from build123d import *

# Parameters (mm, degrees)
SKETCH1_W           = 100
SKETCH1_H           = 30
SKETCH1_R           = 1.5
BOSS_EXTRUDE1_DEPTH = 2
SKETCH2_W           = 1
SKETCH2_H           = 30
BOSS_EXTRUDE3_DEPTH = 50
FILLET2_R           = 1
SKETCH3_R           = 1.5
CUT_EXTRUDE1_DEPTH  = 10
FILLET3_R           = 10
BOSS_EXTRUDE4_DEPTH = 2


with BuildPart() as part:
    # Sketch1 → Boss-Extrude1 (new body)
    with BuildSketch(Plane.XY):
        with Locations((50, 15)):
            Rectangle(SKETCH1_W, SKETCH1_H)
        with Locations((10, 15)):
            Circle(SKETCH1_R, mode=Mode.SUBTRACT)
    extrude(amount=BOSS_EXTRUDE1_DEPTH)

    # Sketch2 → Boss-Extrude3 (add)
    with BuildSketch(Plane.XY.offset(2)):
        with Locations((100.5, 15)):
            Rectangle(SKETCH2_W, SKETCH2_H)
        with Locations((99.5, 15)):
            Rectangle(SKETCH2_W, SKETCH2_H)
    extrude(amount=-BOSS_EXTRUDE3_DEPTH)

    # Fillet2
    fillet2_edges = [part.edges().sort_by_distance(p)[0] for p in [
        (101, 15, 2),
        (99, 15, 0),
    ]]
    fillet(fillet2_edges, radius=FILLET2_R)

    # Sketch3 → Cut-Extrude1 (cut)
    with BuildSketch(Plane(origin=(101, 0, 0), x_dir=(0, 0, -1), z_dir=(1, 0, 0))):
        with Locations(Location((28, 8, 0), (0, 0, 90))):
            Circle(SKETCH3_R)
        with Locations(Location((28, 22, 0), (0, 0, 90))):
            Circle(SKETCH3_R)
    extrude(amount=-CUT_EXTRUDE1_DEPTH, mode=Mode.SUBTRACT)

    # Fillet3
    fillet3_edges = [part.edges().sort_by_distance(p)[0] for p in [
        (100, 0, -48),
        (100, 30, -48),
        (0, 30, 1),
        (0, 0, 1),
    ]]
    fillet(fillet3_edges, radius=FILLET3_R)

    # Sketch4 → Boss-Extrude4 (add)
    with BuildSketch(Plane(origin=(0, 0, 0), x_dir=(1, 0, 0), z_dir=(0, 1, 0))):
        with BuildLine():
            Line((99, 10), (89, 0))
            Line((89, 0), (98, 0))
            ThreePointArc((98, 0), (98.707106781, 0.292893219), (99, 1))
            Line((99, 1), (99, 10))
        make_face()
    boss_extrude4 = extrude(amount=BOSS_EXTRUDE4_DEPTH)

    # Mirror1: Boss-Extrude4 across plane
    add(boss_extrude4.mirror(Plane.ZX.offset(15)))


solid = part.part
Check sheet for the modelled part. Datum: model origin and axes. Units: mm. A direction names the side the tool comes from. Give positions to 0.01 mm unless a question says otherwise; leave off trailing zeros. Write each loop counter-clockwise with the first axis right and the second up, starting at its lowest first coordinate (ties: lowest second). Pieces come first, ordered by that corner, then holes. Notation, with made-up numbers: (45.5, 3.5) -> (73.5, 3.5) arc R17 cw to (73.5, 13.5) -> close; hole circle Ø8 at (-22.75, -8). An arc over 180 degrees is marked (long way). One line per item, written item: value. Start each with the question number.
Item 1: Tool access check on faces 1 (the flat face through (99, 15, -24)), 2 (the cylindrical face through (100.014, 21.805, -26.513)). Record the directions out of +Z, -Z, +X, -X, +Y, -Y that give a thin tool (end or side, any length) a straight path to the whole face; none if there is none.
Item 2: Section check D-D on x = 84.5. Record the cut outline in (y, z), then the cut area to 3 significant figures.
Item 3: Draft check along Y on faces 3 (the flat face through (79, 30, 1)), 4 (the flat face through (96, 2, -3)), 5 (the flat face through (49, 15, 2)), 6 (the flat face through (96, 28, -3)). Enter one of: +Y half, -Y half, draft (parallel to the pull), parting line (faces both ways), or undercut.
Item 4: Section check C-C on z = -22. Record the cut outline in (x, y), then the cut area to 3 significant figures.
Item 5: Material ranges on probe 1 along Y at (x, z) = (10, 1); probe 2 along X at (y, z) = (23, -22); probe 3 along Z at (x, y) = (85, 9.75), recorded low to high. Write a range as from..to.
Item 6: Gauge pin test, flat ends, axial feed: pin 1 (5 mm diameter, centred on x = 10, y = 15, fed in from -Z); pin 2 (3.5 mm diameter, centred on y = 8, z = -28, fed in from -X); pin 3 (5 mm diameter, centred on x = 91.5, z = -3, fed in from +Y). Record the tip position at first contact, or that the pin passes through.
Item 7: Section check A-A on z = -28. Record the cut outline in (x, y), then the cut area to 3 significant figures.
Item 8: Section check B-B on y = 12. Record the cut outline in (x, z).
Results list:
1. face 1: -Z, -X
1. face 2: +X, -X
2. outline: (0, 0) -> (30, 0) -> (30, 2) -> (0, 2) -> close
2. area: 60.0 mm²
3. face 3: +Y half
3. face 4: undercut
3. face 5: draft
3. face 6: undercut
4. outline: (99, 0) -> (101, 0) -> (101, 30) -> (99, 30) -> close
4. area: 60.0 mm²
5. probe 1: 0..13.5, 16.5..30
5. probe 2: 99..101
5. probe 3: 0..2
6. pin 1: z = 0
6. pin 2: x = 99
6. pin 3: y = 30
7. outline: (99, 0) -> (101, 0) -> (101, 6.5) -> (99, 6.5) -> close; (99, 9.5) -> (101, 9.5) -> (101, 20.5) -> (99, 20.5) -> close; (99, 23.5) -> (101, 23.5) -> (101, 30) -> (99, 30) -> close
7. area: 48.0 mm²
8. outline: (0, 0) -> (98, 0) arc R1 cw to (99, -1) -> (99, -48) -> (101, -48) -> (101, 1) arc R1 ccw to (100, 2) -> (0, 2) -> close
